Input: part model. Units: mm. Frame: model coordinates. Face numbers are marked on the shaded views. A direction names the side the tool comes from. Round coordinates to 2 decimals unless told otherwise and drop trailing zeros. Order: outer loops, then holes, each group sorted by start corner. A loop starts at its lowest first (then second) coordinate and runs counter-clockwise, first axis right, second up.
Item 1: Line query: L1, parallel to Z at x = -29.6, y = 7.5; L2, parallel to Z at x = -29, y = 3; L3, parallel to X at y = 11, z = -38.5. Output: solid intervals per line, ascending.
Item 2: First-contact query: pin 1 (12 mm diameter, centred on x = 75.5, z = -19, fed in from -Y); pin 2 (17 mm diameter, centred on y = 35, z = 8.5, fed in from -X); pin 3 (1.2 mm diameter, centred on x = 96.5, z = -43, fed in from -Y); pin 4 (5 mm diameter, centred on x = -95.5, z = 5.5, fed in from +Y). Flat tips, straight axial feed; report the tip coordinate or a pass-through.
Item 3: Cut plane A-A on y = 46.5. Output: boundary loops of the cut face in (x, z).
Item 4: Reachability of the marked faces 1 and 2 from +Z, -Z, +X, -X, +Y, -Y: full face, straight path, thin tool, end or side. Return the list, or none.
Item 5: Cut plane C-C on z = -43. Output: boundary loops of the cut face in (x, y).
Item 6: Cut plane B-B on x = -89. Output: boundary loops of the cut face in (y, z).
Item 7: Mould query, pull axis Z, two halves, no side actions, for the marked faces 3, 4 and 5. Classes: released by +Z, released by -Z, zero draft, split by the parting line, or undercut.
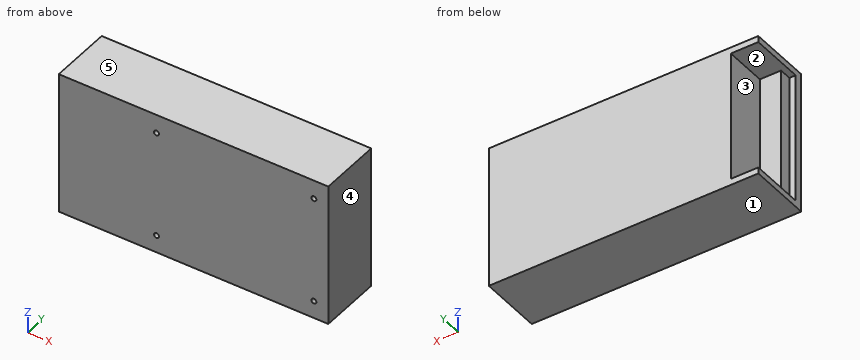
```python
from build123d import *

# Parameters (mm, degrees)
ESBO_O1_W                = 215
ESBO_O1_H                = 114
RESSALTO_EXTRUS_O1_DEPTH = 50
CORTE_EXTRUS_O1_START    = -5
CORTE_EXTRUS_O1_DEPTH    = 104
ESBO_O4_R                = 2
CORTE_EXTRUS_O2_DEPTH    = 10


with BuildPart() as part:
    # Esboço1 → Ressalto-extrusão1 (new body)
    with BuildSketch(Plane(origin=(0, 0, 0), x_dir=(1, 0, 0), z_dir=(0, 1, 0))):
        Rectangle(ESBO_O1_W, ESBO_O1_H)
    extrude(amount=RESSALTO_EXTRUS_O1_DEPTH)

    # Esboço3 → Corte-extrusão1 (cut)
    with BuildSketch(Plane.XY.offset(57).offset(CORTE_EXTRUS_O1_START)):
        Polygon((-107.5, 50), (-85.58523496, 50), (-85.58523496, 16.13389081), (-102.483117777, 16.13389081), (-102.483117777, 6.426889092), (-107.5, 6.426889092), (-107.5, 17.457061978), align=None)
    extrude(amount=-CORTE_EXTRUS_O1_DEPTH, mode=Mode.SUBTRACT)

    # Esboço4 → Corte-extrusão2 (cut)
    with BuildSketch(Plane.XZ):
        with Locations((96, 42)):
            Circle(ESBO_O4_R)
        with Locations((-29.6, 42)):
            Circle(ESBO_O4_R)
        with Locations((-29.6, -43)):
            Circle(ESBO_O4_R)
        with Locations((96, -43)):
            Circle(ESBO_O4_R)
    extrude(amount=-CORTE_EXTRUS_O2_DEPTH, mode=Mode.SUBTRACT)


solid = part.part
```
From the geometry:
1. L1: z = -57 to -45, -41 to 40, 44 to 57
1. L2: z = -57 to -44.91, -41.09 to 40.09, 43.91 to 57
1. L3: x = -102.48 to 107.5
2. pin 1: stops at y = 0
2. pin 2: stops at x = -85.59
2. pin 3: stops at y = 10
2. pin 4: stops at y = 16.13
3. outline: (-107.5, -57) - (107.5, -57) - (107.5, 57) - (-107.5, 57) - (-107.5, 52) - (-85.59, 52) - (-85.59, -52) - (-107.5, -52) - close
4. face 1: -Z, +X, -X, +Y, -Y
4. face 2: -X, +Y
5. outline: (-107.5, 0) - (-31.6, 0) - (-31.6, 10) - (-27.6, 10) - (-27.6, 0) - (94, 0) - (94, 10) - (98, 10) - (98, 0) - (107.5, 0) - (107.5, 50) - (-85.59, 50) - (-85.59, 16.13) - (-102.48, 16.13) - (-102.48, 6.43) - (-107.5, 6.43) - close
6. outline: (0, -57) - (50, -57) - (50, -52) - (16.13, -52) - (16.13, 52) - (50, 52) - (50, 57) - (0, 57) - close
7. face 3: undercut
7. face 4: zero draft
7. face 5: released by +Z
